Can you work these out from the model? Positions are in its coordinate system, mm. A direction names the side the tool comes from. Give positions to 0.01 mm unless a question says otherwise; leave off trailing zeros. Order: outer loops, then holes, each group sorted by start corner. A loop starts at its lowest first (then second) coordinate and runs counter-clockwise, first axis right, second up.
Item 1: If we mould it in two halves opening along X, with no side actions, what happens to faces 6 (the flat face through (4.4, 0, 3)), 7 (the flat face through (1, 1, 5)), 8 (the flat face through (3, -0.9, 4.7))? For each: +X half, -X half, draft (parallel to the pull), parting line (faces both ways), or undercut.
Item 2: Which directions (+Z, -Z, +X, -X, +Y, -Y) give clear straight access to the entire face, cutting with the end or side of a thin tool? Please do faces 1 (the cylindrical face through (0, 4, 6)), 2 (the flat face through (3.5, -0.1, 4)), 3 (the flat face through (0, 4.4, 6.5)), 4 (the flat face through (-3, 0.1, 4.7)), 5 (the flat face through (-4, 0, 0.5)).
Item 3: I want a section at B-B, the plane y = 0. Write out the boundary of the cut face in (x, z).
Item 4: I want a section at A-A, the plane x = 0. Write out the boundary of the cut face in (y, z).
Item 5: I want a section at C-C, the plane z = 2.25. Write out the boundary of the cut face in (x, y).
Item 6: If I drill on line 1 along Y through (x, z) = (0, 1.1); line 2 along X through (y, z) = (0, 3.05), over which ranges is the centre line in solid material (lowest first)?
Item 7: I'm going to push flat-ended pins straight in: pin 1 Ø0.8 at (x, y) = (-4.5, -0.5) entering from -Z; pin 2 Ø2.5 at (x, y) = (-1.5, 3.5) entering from +Z; pin 3 Ø0.5 at (x, y) = (4.5, 1) entering from +Z. Where does each tip first touch, or does it pass through?
Item 8: I want a section at D-D, the plane x = 2.25. Write out the boundary of the cut face in (y, z).
```python
from build123d import *

# Parameters (mm, degrees)
SKETCH2_R           = 5
SKETCH2_R_2         = 1
BOSS_EXTRUDE1_DEPTH = 8
SKETCH3_W           = 1
SKETCH3_H           = 1
SKETCH3_W_2         = 2
SKETCH3_H_2         = 4
CUT_EXTRUDE1_DEPTH  = 4
SKETCH4_R           = 4
CUT_EXTRUDE2_DEPTH  = 3
SKETCH5_W           = 9.370112771
SKETCH5_H           = 5.033531654
CUT_EXTRUDE3_DEPTH  = 1.5


with BuildPart() as part:
    # Sketch2 → Boss-Extrude1 (new body)
    with BuildSketch(Plane.XY):
        Circle(SKETCH2_R)
        Circle(SKETCH2_R_2, mode=Mode.SUBTRACT)
    extrude(amount=BOSS_EXTRUDE1_DEPTH)

    # Sketch3 → Cut-Extrude1 (cut, symmetric)
    with BuildSketch(Plane(origin=(0, 0, 0), x_dir=(1, 0, 0), z_dir=(0, 1, 0))):
        with Locations((-4.5, -0.5)):
            Rectangle(SKETCH3_W, SKETCH3_H)
        Polygon((5, -8), (3, -8), (3, -4), (4, -4), (4, -3), (5, -3), align=None)
        with Locations((-4, -6)):
            Rectangle(SKETCH3_W_2, SKETCH3_H_2)
    extrude(amount=CUT_EXTRUDE1_DEPTH, both=True, mode=Mode.SUBTRACT)

    # Sketch4 → Cut-Extrude2 (cut)
    with BuildSketch(Plane.XY.offset(8)):
        Circle(SKETCH4_R)
    extrude(amount=-CUT_EXTRUDE2_DEPTH, mode=Mode.SUBTRACT)

    # Sketch5 → Cut-Extrude3 (cut)
    with BuildSketch(Plane.XY.offset(8)):
        with Locations((0.643727428, 3.756174823)):
            Rectangle(SKETCH5_W, SKETCH5_H)
    extrude(amount=-CUT_EXTRUDE3_DEPTH, mode=Mode.SUBTRACT)


solid = part.part
```
Results list:
1. face 6: draft
1. face 7: undercut
1. face 8: +X half
2. face 1: +Z
2. face 2: +Z, +X, +Y, -Y
2. face 3: +Z, +X, -X, +Y
2. face 4: +Z, -X, +Y, -Y
2. face 5: -Z, -X, +Y, -Y
3. outline: (-5, 1) - (-4, 1) - (-4, 0) - (-1, 0) - (-1, 5) - (-3, 5) - (-3, 4) - (-5, 4) - close; (1, 0) - (5, 0) - (5, 3) - (4, 3) - (4, 4) - (3, 4) - (3, 5) - (1, 5) - close
4. outline: (-5, 0) - (-1, 0) - (-1, 5) - (-4, 5) - (-4, 8) - (-5, 8) - close; (1, 0) - (5, 0) - (5, 6.5) - (4, 6.5) - (4, 5) - (1, 5) - close
5. outline: circle Ø10 at (0, 0); hole circle Ø2 at (0, 0)
6. line 1: y = -5 to -1, 1 to 5
6. line 2: x = -5 to -1, 1 to 4
7. pin 1: stops at z = 1
7. pin 2: stops at z = 6.5
7. pin 3: stops at z = 3
8. outline: (-4.47, 0) - (4.47, 0) - (4.47, 6.5) - (3.31, 6.5) - (3.31, 5) - (-3.31, 5) - (-3.31, 8) - (-4.47, 8) - close
